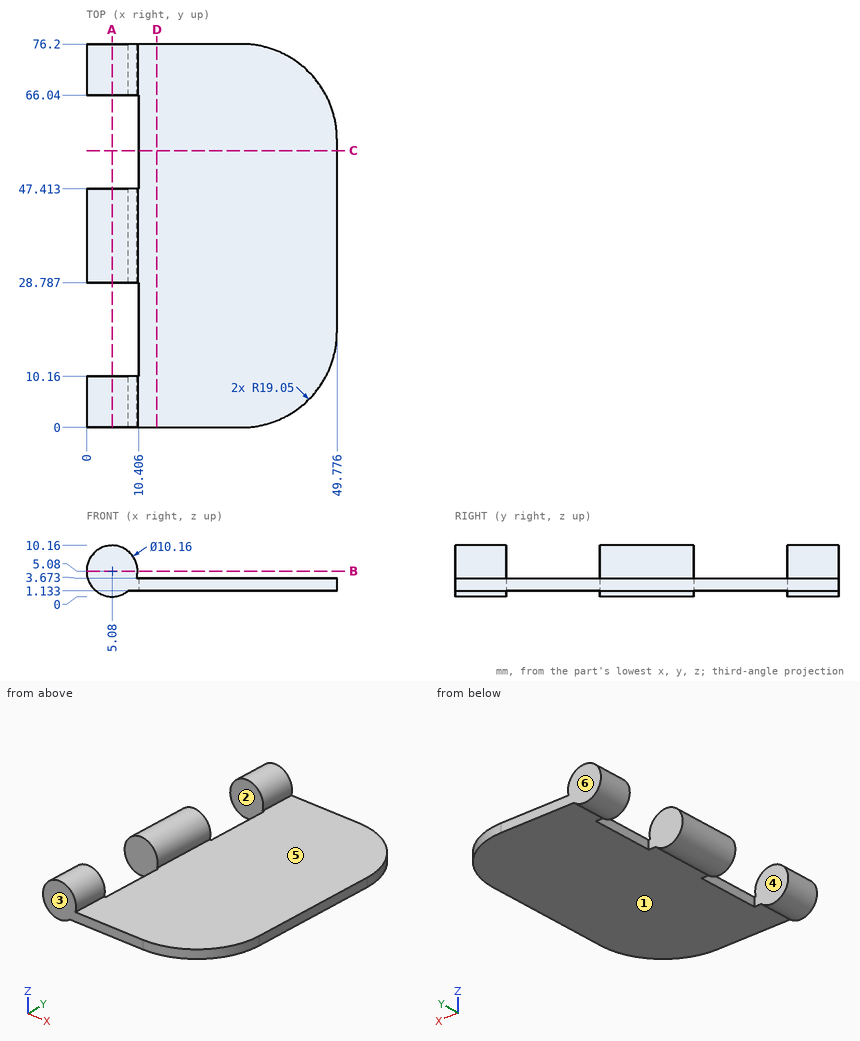
Check sheet for the drawn part. Datum: minimum x, y, z corner. Units: mm. A direction names the side the tool comes from. Round coordinates to 2 decimals unless told otherwise and drop trailing zeros. Write each loop counter-clockwise with the first axis right and the second up, starting at its lowest first coordinate (ties: lowest second). Pieces come first, ordered by that corner, then holes. Notation, with made-up numbers: (-25, -6.75) -> (3, -6.75) arc R16 cw to (3, 18.25) -> close; hole circle Ø4 at (57.5, -35.75). An arc over 180 degrees is marked (long way). One line per item, written item: value. Start each with the question number.
(1) Draft check along Y on the marked faces 4, 5 and 6. Enter one of: +Y half, -Y half, draft (parallel to the pull), parting line (faces both ways), or undercut.
(2) Cross-section at B-B, the plane z = 5.08. Record the cut outline in (x, y), and give its area (3 significant figures).
(3) Go/stop test with flat-tipped pins: pin 1 Ø5 at (x, y) = (28, 33.5) entering from -Z; pin 2 Ø1.5 at (x, y) = (32, 31.5) entering from +Z; pin 3 Ø0.8 at (y, z) = (16, 3) entering from -X; pin 4 Ø3 at (x, z) = (7, 5) entering from -Y. Record where each tip stops, or that it passes through.
(4) Cross-section at D-D, the plane x = 14. Record the cut outline in (y, z).
(5) Cross-section at A-A, the plane x = 5.08. Record the cut outline in (y, z), and give its area (3 significant figures).
(6) Scan lines: line 1 (Y direction, x = 3, z = 3.5); line 2 (Z direction, x = 29, y = 5); line 3 (X direction, y = 33, z = 5.5). Record each from-to range of solid material in increasing order. Write a range as [from, to].
(7) Cross-section at C-C, the plane y = 55. Record the cut outline in (x, z).
(8) Access from +Z, -Z, +X, -X, +Y, -Y to the whole of each face (thin tool, end or side, straight path). Record for the marked faces 1, 2 and 3.
Answer:
1. face 4: undercut
1. face 5: draft
1. face 6: +Y half
2. outline: (0, 0) -> (10.16, 0) -> (10.16, 10.16) -> (0, 10.16) -> close; (0, 28.79) -> (10.16, 28.79) -> (10.16, 47.41) -> (0, 47.41) -> close; (0, 66.04) -> (10.16, 66.04) -> (10.16, 76.2) -> (0, 76.2) -> close
2. area: 396 mm²
3. pin 1: z = 1.13
3. pin 2: z = 3.67
3. pin 3: x = 10.41
3. pin 4: y = 0
4. outline: (0, 1.13) -> (76.2, 1.13) -> (76.2, 3.67) -> (0, 3.67) -> close
5. outline: (0, 0) -> (10.16, 0) -> (10.16, 10.16) -> (0, 10.16) -> close; (28.79, 0) -> (47.41, 0) -> (47.41, 10.16) -> (28.79, 10.16) -> close; (66.04, 0) -> (76.2, 0) -> (76.2, 10.16) -> (66.04, 10.16) -> close
5. area: 396 mm²
6. line 1: [0, 10.16], [28.79, 47.41], [66.04, 76.2]
6. line 2: [1.13, 3.67]
6. line 3: [0.02, 10.14]
7. outline: (10.41, 1.13) -> (49.78, 1.13) -> (49.78, 3.67) -> (10.41, 3.67) -> close
8. face 1: -Z, +X, +Y, -Y
8. face 2: +Z, -Z, -X
8. face 3: +Z, -Z, +X, -X, -Y
